Read the model definition and answer for the solid it produces. Units are mm, in the model's axes. Face numbers are marked on the shaded views. A direction names the side the tool comes from. Coordinates: 2 decimals unless noted, no trailing zeros. Order: outer loops, then holes, each group sorted by start corner. A loop starts at its lowest first (then second) coordinate and runs counter-clockwise, first axis right, second up. Notation, with made-up numbers: (81, 17) - (134, 17) arc R36 ccw to (134, 54) - close; hole circle Ø5 at (61.5, -5). An arc over 180 degrees is marked (long way). Use one line per item in the form item = value. Start each with the question number.
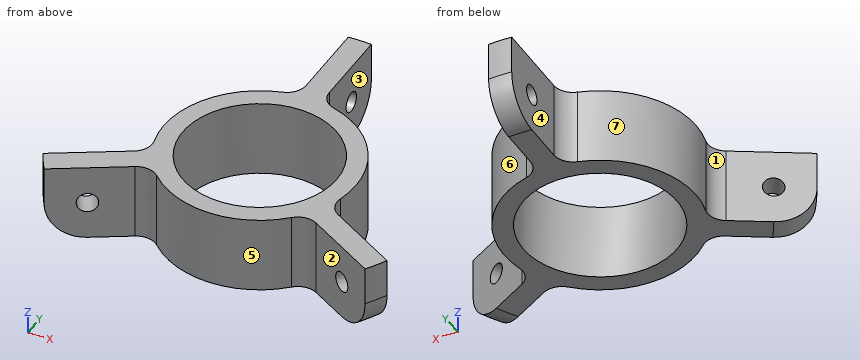
from build123d import *

# Parameters (mm, degrees)
SKETCH_R              = 50
SKETCH_R_2            = 20
PAD_DEPTH             = 20
POCKET_DEPTH          = 305.658137
POLARPATTERN_COUNT    = 3
SKETCH003_R           = 2.6
POCKET002_DEPTH       = 287.850495
POLARPATTERN001_COUNT = 3
FILLET_R              = 5
FILLET001_R           = 10


with BuildPart() as part:
    # Sketch → Pad (new body)
    with BuildSketch(Plane.XY):
        Circle(SKETCH_R)
        Circle(SKETCH_R_2, mode=Mode.SUBTRACT)
    extrude(amount=PAD_DEPTH)

    # Sketch001 (on Face4 of Pad) → Pocket (cut, through all)
    with BuildSketch(Plane.XY.offset(20)):
        with BuildLine():
            ThreePointArc((22.994185, -9.811597), (21.650635, 12.5), (3, 24.819347))
            Line((3, 55.952225), (3, 24.819347))
            ThreePointArc((49.956048, -25.378036), (48.525649, 28.016297), (3, 55.952225))
            Line((22.994185, -9.811597), (49.956048, -25.378036))
        make_face()
    pocket = extrude(amount=-POCKET_DEPTH, mode=Mode.SUBTRACT)

    # PolarPattern: Pocket ×3 about axis
    polarpattern_axis = Axis((0, 0, 20), (0, 0, 1))
    for i in range(1, POLARPATTERN_COUNT):
        add(pocket.rotate(polarpattern_axis, i * 360 / POLARPATTERN_COUNT), mode=Mode.SUBTRACT)

    # Sketch003 → Pocket002 (cut, through all)
    with BuildSketch(Plane.YZ.offset(3)):
        with Locations((39.909919, 10)):
            Circle(SKETCH003_R)
    pocket002 = extrude(amount=-POCKET002_DEPTH, mode=Mode.SUBTRACT)

    # PolarPattern001: Pocket002 ×3 about axis
    polarpattern001_axis = Axis((0, 0, 0), (0, 0, 1))
    for i in range(1, POLARPATTERN001_COUNT):
        add(pocket002.rotate(polarpattern001_axis, i * 360 / POLARPATTERN001_COUNT), mode=Mode.SUBTRACT)

    # Fillet
    fillet_edges = [part.edges().sort_by_distance(p)[0] for p in [
        (-22.994185, -9.811597, 10),
        (-19.994185, -15.00775, 10),
        (19.994185, -15.00775, 10),
        (22.994185, -9.811597, 10),
        (3, 24.819347, 10),
        (-3, 24.819347, 10),
    ]]
    fillet(fillet_edges, radius=FILLET_R)

    # Fillet001
    fillet001_edges = [part.edges().sort_by_distance(p)[0] for p in [
        (0, 50, 0),
        (-43.30127, -25, 0),
        (43.30127, -25, 0),
    ]]
    fillet(fillet001_edges, radius=FILLET001_R)


solid = part.part
Q1. For a pull along X with two mould halves and no side action, classify the marked faces 5, 6 and 7 as +X half, -X half, draft (parallel to the pull), parting line (faces both ways), or undercut.
Q2. A cutting plane is placed at A-A (x = 0). Give the vertices of the cut face in (y, z).
Q3. Which of the six approach directions +Z, -Z, +X, -X, +Y, -Y give full straight-line access (tool end or side, diameter ignored) to the marked faces 1, 2, 3 and 4?
Q4. Consider probe 1 along X at (y, z) = (-21, 14.25); probe 2 along X at (y, z) = (35, 16); probe 3 along Y at (x, z) = (-2, 5). Determine where each line is inside the solid, lowest interval first.
Q5. A cutting plane is placed at B-B (y = 0). Give the vertices of the cut face in (x, z), then the cut area to 3 significant figures.
Q6. A cutting plane is placed at C-C (z = 11.5). Give the number of separate pieces and of enclosed holes in the cut face, then the cut area to 3 significant figures.
Q7. A cutting plane is placed at D-D (x = 19). Give the vertices of the cut face in (y, z) (3 decimals), then the cut area to 3 significant figures.
Q8. Given P1, Ø5, axis at x = -24, z = 13, coming from the +Y side; P2, Ø1.5, axis at x = 10, z = 12.5, coming from the -Y side; P3, Ø10, axis at x = 35, z = 14, coming from the -Y side, each flat-ended and moving along its own axis, determine where each tip first touches the part or whether it passes through.
Result sheet:
q1.face_5 = undercut
q1.face_6 = +X half
q1.face_7 = -X half
q2.outline = (-25, 0) - (-20, 0) - (-20, 20) - (-25, 20) - close; (20, 0) - (40, 0) arc R10 ccw to (50, 10) - (50, 20) - (20, 20) - close; hole circle Ø5.2 at (39.91, 10)
q3.face_1 = +Z, -Z, -X
q3.face_2 = +Z, -Z, -Y
q3.face_3 = +Z, -Z, +X, +Y
q3.face_4 = +Z, -Z, -X, +Y
q4.probe_1 = -42.37 to -30.37, -13.56 to 13.56, 30.37 to 42.37
q4.probe_2 = -3 to 3
q4.probe_3 = -24.92 to -19.9, 19.9 to 48.62
q5.outline = (-25, 0) - (-20, 0) - (-20, 20) - (-25, 20) - close; (20, 0) - (25, 0) - (25, 20) - (20, 20) - close
q5.area = 200 mm^2
q6.separate_pieces = 4
q6.enclosed_holes = 1
q6.area = 1,100 mm^2
q7.outline = (-16.82, 0) - (-6.245, 0) - (-6.245, 20) - (-16.82, 20) - close; (6.245, 0) - (16.248, 0) - (16.248, 20) - (6.245, 20) - close
q7.area = 412 mm^2
q8.P1 = 12.76
q8.P2 = -23.23
q8.P3 = -26.56
